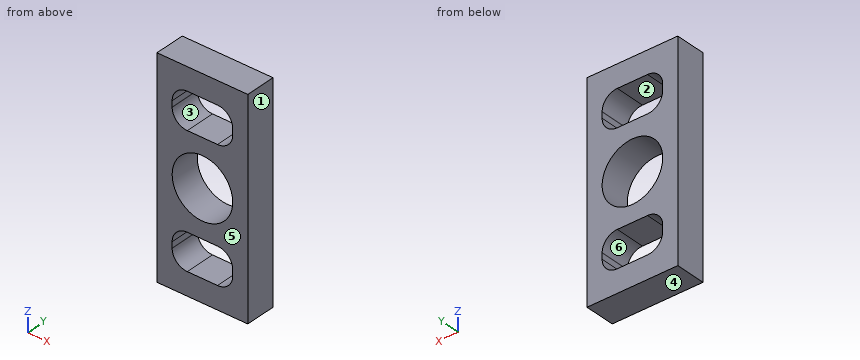
```python
from build123d import *

# Parameters (mm, degrees)
SKETCH1_W           = 38.1
SKETCH1_H           = 12.7
BOSS_EXTRUDE1_DEPTH = 88.9
SKETCH2_R           = 12.7
CUT_EXTRUDE1_DEPTH  = 88.9
SKETCH3_W           = 25.4
SKETCH3_H           = 15.24
CUT_EXTRUDE2_DEPTH  = 12.7
FILLET1_R           = 6.35


with BuildPart() as part:
    # Sketch1 → Boss-Extrude1 (new body)
    with BuildSketch(Plane.XY):
        with Locations((-5.693103448, -0.218965517)):
            Rectangle(SKETCH1_W, SKETCH1_H)
    extrude(amount=BOSS_EXTRUDE1_DEPTH)

    # Sketch2 → Cut-Extrude1 (cut)
    with BuildSketch(Plane(origin=(0, 6.131034483, 0), x_dir=(1, 0, 0), z_dir=(0, 1, 0))):
        with Locations(Location((-5.693103448, -44.45, 0), (0, 0, 180))):
            Circle(SKETCH2_R)
    extrude(amount=-CUT_EXTRUDE1_DEPTH, mode=Mode.SUBTRACT)

    # Sketch3 → Cut-Extrude2 (cut)
    with BuildSketch(Plane(origin=(0, 6.131034483, 0), x_dir=(1, 0, 0), z_dir=(0, 1, 0))):
        with Locations((-5.693103448, -17.145)):
            Rectangle(SKETCH3_W, SKETCH3_H)
        with Locations((-5.693103448, -71.755)):
            Rectangle(SKETCH3_W, SKETCH3_H)
    extrude(amount=-CUT_EXTRUDE2_DEPTH, mode=Mode.SUBTRACT)

    # Fillet1
    fillet1_edges = [part.edges().sort_by_distance(p)[0] for p in [
        (-18.393103448, -0.218965517, 24.765),
        (-18.393103448, -0.218965517, 9.525),
        (7.006896552, -0.218965517, 9.525),
        (7.006896552, -0.218965517, 24.765),
        (-18.393103448, -0.218965517, 79.375),
        (-18.393103448, -0.218965517, 64.135),
        (7.006896552, -0.218965517, 64.135),
        (7.006896552, -0.218965517, 79.375),
    ]]
    fillet(fillet1_edges, radius=FILLET1_R)


solid = part.part
```
For this review, take the finished solid that the model builds, in its own axes (mm). Face numbers are marked on the shaded views. A direction names the side the tool comes from. Give positions to 0.01 mm unless a question says otherwise; leave off trailing zeros. Write each loop counter-clockwise with the first axis right and the second up, starting at its lowest first coordinate (ties: lowest second). Pieces come first, ordered by that corner, then holes. Notation, with made-up numbers: M 34,88 L 79,88 A32 cw 79,127 Z; hole C 67,46.5 d4. An arc over 180 degrees is marked long. Answer as a JSON object with one key per item and string values. Group by question number.
Item 1: Consider section D-D on x = -6. Write out the cut boundary in (y, z) (3 decimals), plus the area to 3 significant figures.
Item 2: Consider section C-C on x = -13. Write out the cut boundary in (y, z).
Item 3: Tool access review of the marked faces 5 and 6: name each direction out of +Z, -Z, +X, -X, +Y, -Y from which nothing blocks a thin tool from reaching the whole face with its end or side.
Item 4: Consider section A-A on z = 44.45. Write out the cut boundary in (x, y), plus the area to 3 significant figures.
Item 5: For pin 1 Ø20.5 at (x, z) = (-5.69, 44.45) entering from -Y, flat-tipped, find the tip position at first contact; note if it passes through.
Item 6: Draft analysis for pull direction Z (two halves, no side actions). For the marked faces 1, 2, 3 and 4, state which applies: +Z half, -Z half, draft (parallel to the pull), parting line (faces both ways), or undercut.
Item 7: For probe 1 along Z at (x, y) = (-8, -2) (3 decimals); probe 2 along Z at (x, y) = (3.5, 4.5); probe 3 along X at (y, z) = (1, 16), list the stretches that pass through material, from the lowest coordinate up. Write a range as [from, to].
Item 8: Consider section B-B on y = -2. Write out the cut boundary in (x, z) (3 decimals), plus the area to 3 significant figures.
Check result:
{
 "1": {"outline": "M -6.569,0 L 6.131,0 L 6.131,9.525 L -6.569,9.525 Z; M -6.569,24.765 L 6.131,24.765 L 6.131,31.754 L -6.569,31.754 Z; M -6.569,57.146 L 6.131,57.146 L 6.131,64.135 L -6.569,64.135 Z; M -6.569,79.375 L 6.131,79.375 L 6.131,88.9 L -6.569,88.9 Z", "area": "419 mm^2"},
 "2": {"outline": "M -6.57,0 L 6.13,0 L 6.13,9.6 L -6.57,9.6 Z; M -6.57,24.69 L 6.13,24.69 L 6.13,34.06 L -6.57,34.06 Z; M -6.57,54.84 L 6.13,54.84 L 6.13,64.21 L -6.57,64.21 Z; M -6.57,79.3 L 6.13,79.3 L 6.13,88.9 L -6.57,88.9 Z"},
 "3": {"face 5": "+Z, -Z, +X, -X, -Y", "face 6": "+Y, -Y"},
 "4": {"outline": "M -24.74,-6.57 L -18.39,-6.57 L -18.39,6.13 L -24.74,6.13 Z; M 7.01,-6.57 L 13.36,-6.57 L 13.36,6.13 L 7.01,6.13 Z", "area": "161 mm^2"},
 "5": {"pin 1": "passes through"},
 "6": {"face 1": "draft", "face 2": "undercut", "face 3": "undercut", "face 4": "-Z half"},
 "7": {"probe 1": "z = [0, 9.525], [24.765, 31.961], [56.939, 64.135], [79.375, 88.9]", "probe 2": "z = [0, 10.2], [24.09, 35.69], [53.21, 64.81], [78.7, 88.9]", "probe 3": "x = [-24.74, -18.39], [7.01, 13.36]"},
 "8": {"outline": "M -24.743,0 L 13.357,0 L 13.357,88.9 L -24.743,88.9 Z; hole M -18.393,15.875 A6.35 ccw -12.043,9.525 L 0.657,9.525 A6.35 ccw 7.007,15.875 L 7.007,18.415 A6.35 ccw 0.657,24.765 L -12.043,24.765 A6.35 ccw -18.393,18.415 Z; hole C -5.693,44.45 d25.4; hole M -18.393,70.485 A6.35 ccw -12.043,64.135 L 0.657,64.135 A6.35 ccw 7.007,70.485 L 7.007,73.025 A6.35 ccw 0.657,79.375 L -12.043,79.375 A6.35 ccw -18.393,73.025 Z", "area": "2,180 mm^2"}
}
